The listing builds one solid part. Answer for the finished solid, in the listing's coordinates (mm). A direction names the side the tool comes from. Give positions to 0.01 mm unless a question says otherwise; leave off trailing zeros. Loops run counter-clockwise (first coordinate to the right, second up) from the corner with the lowest first, then second, coordinate; pieces in that order, holes last. Notation, with made-up numbers: (-4.75, 1) - (41.25, 1) arc R36 ccw to (41.25, 38) - close; hole circle Ø8 at (-0.75, 39). An arc over 180 degrees is marked (long way). Answer as CSV lines item,"result". Start each with the question number.
1) Flat-ended cylindrical pins translate along their axes: pin 1 (10 mm diameter, centred on x = -287, z = -157.5, fed in from -Y); pin 2 (10 mm diameter, centred on x = -292.5, z = 174.5, fed in from -Y). Find the tip coordinate at first contact, or state that the pin passes through.
2) For a pull along X with two mould halves and no side action, classify faces 1 (the face through (-24, 400, 216)), 2 (the face through (-4, 197, -205)), 3 (the face through (-300, 203, -3)) as pulls with the +X half, pulls with the -X half, needs draft (parallel to the pull), parting line crosses it, or undercut.
3) Find the intervals of material crossed by line 1 along Z through (x, y) = (40, 145.5); line 2 along X through (y, z) = (46.5, 186); line 3 along Y through (x, z) = (157.5, -166.5), in increasing order.
4) A cutting plane is placed at C-C (z = -33.5). Determine the outline of the cut face in (x, y), and give its area (3 significant figures).
5) For faces 4 (the face through (-290, 160, -156)), 5 (the face through (300, 203, -3)), 6 (the face through (-280, 197, 3)), determine the directions among +Z, -Z, +X, -X, +Y, -Y from which every point of the face is accessible in a straight line to the end or side of a thin tool.
6) A cutting plane is placed at A-A (y = 221). Determine the outline of the cut face in (x, z), and give its area (3 significant figures).
7) A cutting plane is placed at B-B (z = -173). Determine the outline of the cut face in (x, y).
8) A cutting plane is placed at D-D (x = -196.5). Determine the outline of the cut face in (y, z), and give its area (3 significant figures).
```python
from build123d import *

# Parameters (mm, degrees)
SKETCH1_W           = 600
SKETCH1_H           = 450
SKETCH1_W_2         = 560
SKETCH1_H_2         = 410
BOSS_EXTRUDE1_DEPTH = 400
SKETCH2_W           = 600
SKETCH2_H           = 450
BOSS_EXTRUDE2_DEPTH = 20
FILLET1_R           = 20
SKETCH8_W           = 80
SKETCH8_H           = 80
CUT_EXTRUDE3_DEPTH  = 20


with BuildPart() as part:
    # Sketch1 → Boss-Extrude1 (new body)
    with BuildSketch(Plane(origin=(0, 0, 0), x_dir=(1, 0, 0), z_dir=(0, 1, 0))):
        Rectangle(SKETCH1_W, SKETCH1_H)
        Rectangle(SKETCH1_W_2, SKETCH1_H_2, mode=Mode.SUBTRACT)
    extrude(amount=BOSS_EXTRUDE1_DEPTH)

    # Sketch2 → Boss-Extrude2 (add)
    with BuildSketch(Plane.XZ):
        Rectangle(SKETCH2_W, SKETCH2_H)
    extrude(amount=BOSS_EXTRUDE2_DEPTH)

    # Fillet1
    fillet1_edges = [part.edges().sort_by_distance(p)[0] for p in [
        (300, -20, 0),
        (0, -20, 225),
        (-300, -20, 0),
        (0, -20, -225),
    ]]
    fillet(fillet1_edges, radius=FILLET1_R)

    # Sketch8 → Cut-Extrude3 (cut)
    with BuildSketch(Plane.ZY.offset(300)):
        with Locations((155, 200)):
            Rectangle(SKETCH8_W, SKETCH8_H)
        with Locations((-155, 200)):
            Rectangle(SKETCH8_W, SKETCH8_H)
    extrude(amount=-CUT_EXTRUDE3_DEPTH, mode=Mode.SUBTRACT)


solid = part.part
```
Ans:
1,pin 1,"y = -19.9"
1,pin 2,"y = -18.54"
2,face 1,"needs draft"
2,face 2,"undercut"
2,face 3,"pulls with the -X half"
3,line 1,"-225 to -205, 205 to 225"
3,line 2,"-300 to -280, 280 to 300"
3,line 3,"-20 to 0"
4,outline,"(-300, 0) arc R20 ccw to (-280, -20) - (280, -20) arc R20 ccw to (300, 0) - (300, 400) - (280, 400) - (280, 0) - (-280, 0) - (-280, 400) - (-300, 400) - close"
4,area,"27,800 mm2"
5,face 4,"-X"
5,face 5,"+Z, -Z, +X, +Y, -Y"
5,face 6,"+Y"
6,outline,"(-300, -225) - (300, -225) - (300, 225) - (-300, 225) - (-300, 195) - (-280, 195) - (-280, 205) - (280, 205) - (280, -205) - (-280, -205) - (-280, -195) - (-300, -195) - close; (-300, -115) - (-280, -115) - (-280, 115) - (-300, 115) - close"
6,area,"37,200 mm2"
7,outline,"(-300, 0) arc R20 ccw to (-280, -20) - (280, -20) arc R20 ccw to (300, 0) - (300, 400) - (280, 400) - (280, 0) - (-280, 0) - (-280, 160) - (-300, 160) - close; (-300, 240) - (-280, 240) - (-280, 400) - (-300, 400) - close"
8,outline,"(-20, -205) arc R20 ccw to (0, -225) - (400, -225) - (400, -205) - (0, -205) - (0, 205) - (400, 205) - (400, 225) - (0, 225) arc R20 ccw to (-20, 205) - close"
8,area,"24,800 mm2"
